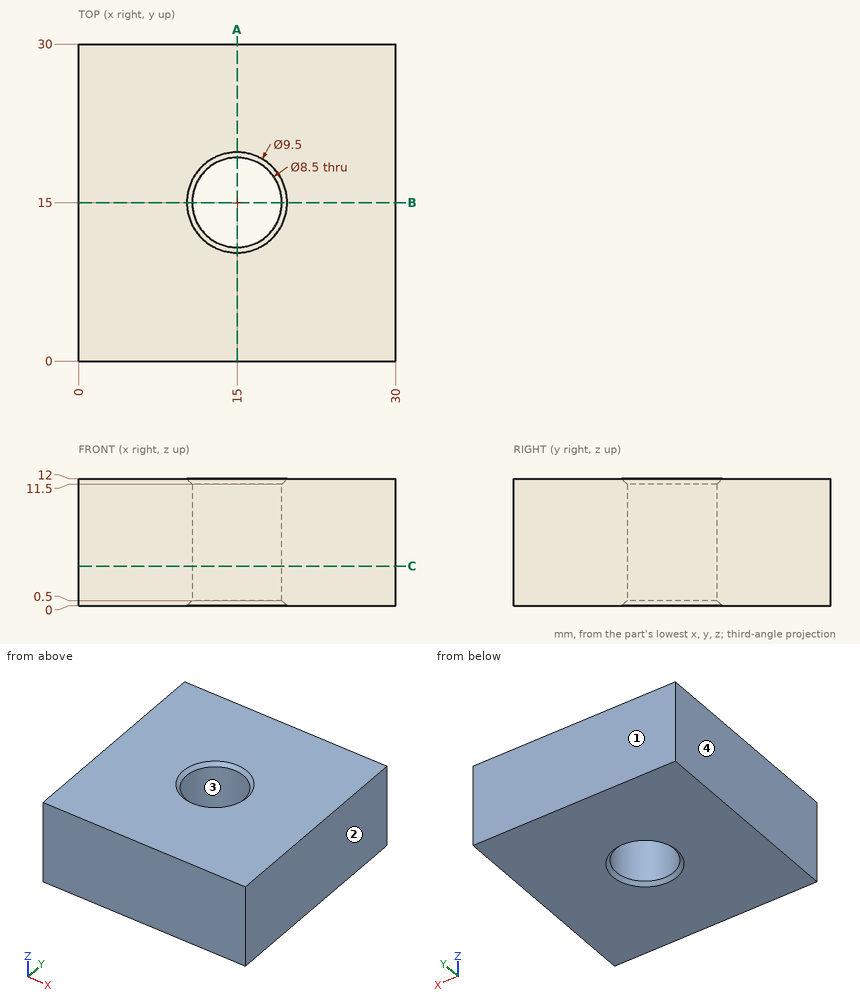
Input: dimensioned drawing with shaded views. Units: mm. Origin: part minimum x, y, z. Give positions to 0.01 mm unless a question says otherwise; leave off trailing zeros. Write each loop counter-clockwise with the first axis right and the second up, starting at its lowest first coordinate (ties: lowest second). Pieces come first, ordered by that corner, then holes. Notation, with made-up numbers: (-9, 17.5) -> (-2, 17.5) arc R13 ccw to (-2, 35.5) -> close; hole circle Ø2 at (17, -6.75). An arc over 180 degrees is marked (long way). Return JSON: item names as keys, results as strings. Group by question number.
1. Mould query, pull axis X, two halves, no side actions, for the marked faces 1, 2, 3 and 4. Classes: +X half, -X half, draft (parallel to the pull), parting line (faces both ways), or undercut.
2. Section A-A, the plane x = 15. Output: boundary loops of the cut face in (y, z).
3. Material intervals for line 1 (Y direction, x = 15, z = 5.25); line 2 (Y direction, x = 13.75, z = 11.75); line 3 (X direction, y = 11.75, z = 3.25), sorted ascending. Write a range as from..to.
4. Section C-C, the plane z = 3.75. Output: boundary loops of the cut face in (x, y), then the cut area to 3 significant figures.
Determined:
{
 "1": {"face 1": "draft", "face 2": "+X half", "face 3": "undercut", "face 4": "-X half"},
 "2": {"outline": "(0, 0) -> (10.25, 0) -> (10.75, 0.5) -> (10.75, 11.5) -> (10.25, 12) -> (0, 12) -> close; (19.25, 0.5) -> (19.75, 0) -> (30, 0) -> (30, 12) -> (19.75, 12) -> (19.25, 11.5) -> close"},
 "3": {"line 1": "y = 0..10.75, 19.25..30", "line 2": "y = 0..10.68, 19.32..30", "line 3": "x = 0..12.26, 17.74..30"},
 "4": {"outline": "(0, 0) -> (30, 0) -> (30, 30) -> (0, 30) -> close; hole circle Ø8.5 at (15, 15)", "area": "843 mm2"}
}
